Answer from the drawing. Dimensions are ordinates in mm from the lowest x, y and z of the part. A direction names the side the tool comes from. Give positions to 0.01 mm unless a question says otherwise; leave off trailing zeros. Write each loop counter-clockwise with the first axis right and the second up, starting at its lowest first coordinate (ties: lowest second). Pieces come first, ordered by that corner, then holes. Notation, with made-up numbers: M 9,38.5 L 26,38.5 A8 cw 26,45.5 Z; hole C -16.75,-32 d10. An arc over 180 degrees is marked long. Write each question's results on one line, items separated by ' | '. Start each with the question number.
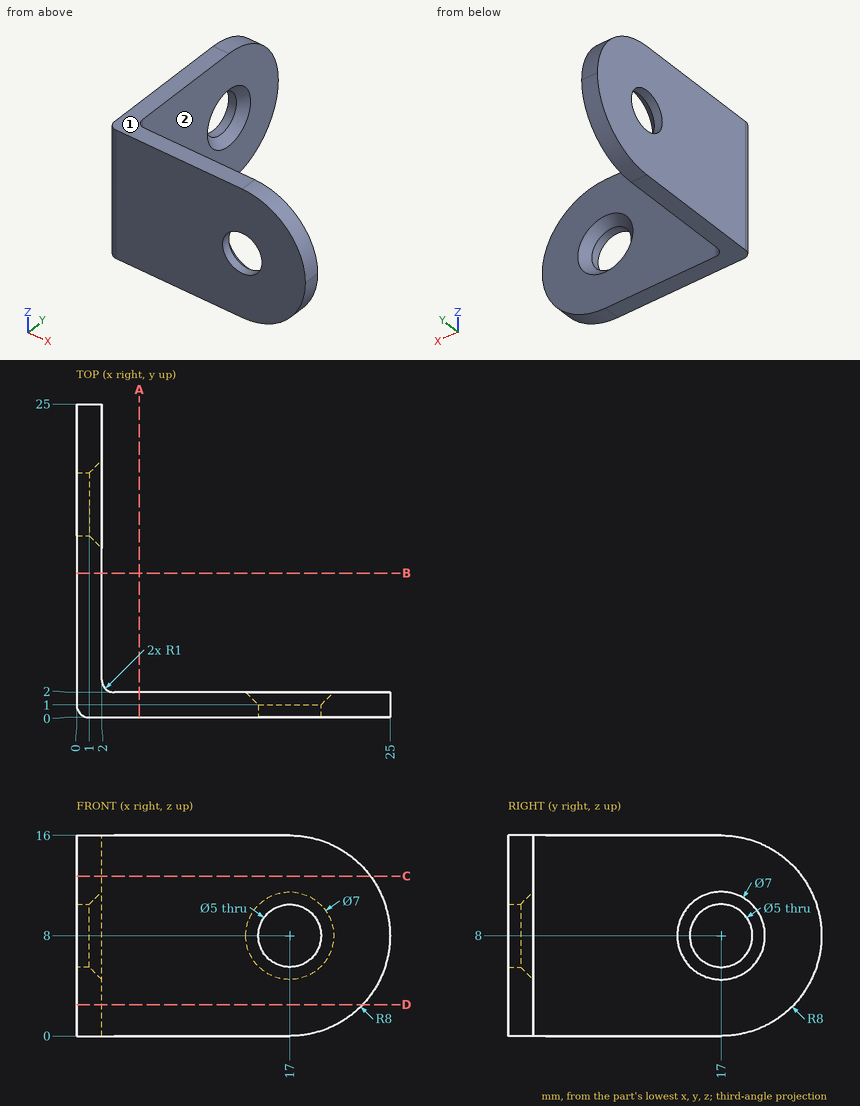
Item 1: Section C-C, the plane z = 12.75 is taken. Determine the outline of the cut face in (x, y).
Item 2: Section D-D, the plane z = 2.5 is taken. Determine the outline of the cut face in (x, y).
Item 3: For the marked faces 1 and 2, determine the directions among +Z, -Z, +X, -X, +Y, -Y from which every point of the face is accessible in a straight line to the end or side of a thin tool.
Item 4: Given P1, Ø6, axis at x = 17, z = 8, coming from the +Y side; P2, Ø1, axis at y = 22, z = 10, coming from the +X side; P3, Ø5, axis at x = 19, z = 7.5, coming from the +Y side, each flat-ended and moving along its own axis, determine where each tip first touches the part or whether it passes through.
Item 5: Straight lines are drawn through the part: line 1 (Z direction, x = 17, y = 0.6); line 2 (X direction, y = 10.25, z = 7.5). For each, find the intervals that lie inside material, in ascending order.
Item 6: Section A-A, the plane x = 5 is taken. Determine the outline of the cut face in (y, z).
Worked out:
1) outline: M 0,1 A1 ccw 1,0 L 23.44,0 L 23.44,2 L 3,2 A1 cw 2,3 L 2,23.44 L 0,23.44 Z
2) outline: M 0,1 A1 ccw 1,0 L 22.81,0 L 22.81,2 L 3,2 A1 cw 2,3 L 2,22.81 L 0,22.81 Z
3) face 1: +Z, +X, -X, +Y, -Y | face 2: +Z, -Z, +X, +Y
4) P1: stops at y = 1.5 | P2: stops at x = 2 | P3: stops at y = 2
5) line 1: z = 0 to 5.5, 10.5 to 16 | line 2: x = 0 to 2
6) outline: M 0,0 L 2,0 L 2,16 L 0,16 Z
